Source: CAD feature listing. Evaluate the final solid. Frame: model axes, mm. A direction names the side the tool comes from. Coordinates: 2 decimals unless noted, no trailing zeros. Order: outer loops, then holes, each group sorted by start corner. A loop starts at its lowest first (then second) coordinate and runs counter-clockwise, first axis right, second up.
```python
from build123d import *

# Parameters (mm, degrees)
GEH_USEKORPUS_DEPTH                = 12.5
GEH_USEAUSH_HLUNG_DEPTH            = 10.5
PLATINENHALTERUNG_DEPTH            = 4.7
SKETCH8_R                          = 1.1
SCHRAUBL_CHER_DEPTH                = 43.096199353
SCHRAUBENMUTTER_AUSNEHMUNGEN_DEPTH = 3
SKETCH10_R                         = 3.25
SKETCH10_R_2                       = 2
BUTTON_AUSNEHMUNGEN_DEPTH          = 3
SCHNITT_LINEAR_AUSTRAGEN1_DEPTH    = 10
SKIZZE2_W                          = 52.65
SKIZZE2_H                          = 1.75
SCHNITT_LINEAR_AUSTRAGEN2_DEPTH    = 1.5
SKIZZE3_W                          = 6
SKIZZE3_H                          = 1
SCHNITT_LINEAR_AUSTRAGEN3_DEPTH    = 1.5
VERRUNDUNG1_R                      = 0.5
VERRUNDUNG2_R                      = 1


with BuildPart() as part:
    # Sketch1 → Gehäusekorpus (new body)
    with BuildSketch(Plane.XY):
        with BuildLine():
            Line((-27, -29.5), (27, -29.5))
            ThreePointArc((27, -29.5), (28.414213562, -28.914213562), (29, -27.5))
            Line((29, -27.5), (29, 27.5))
            ThreePointArc((29, 27.5), (28.414213562, 28.914213562), (27, 29.5))
            Line((27, 29.5), (-27, 29.5))
            ThreePointArc((-27, 29.5), (-28.414213562, 28.914213562), (-29, 27.5))
            Line((-29, 27.5), (-29, -27.5))
            ThreePointArc((-29, -27.5), (-28.414213562, -28.914213562), (-27, -29.5))
        make_face()
    extrude(amount=GEH_USEKORPUS_DEPTH)

    # Sketch3 → Gehäuseaushöhlung (cut)
    with BuildSketch(Plane.XY.offset(12.5)):
        with BuildLine():
            Line((-25.1, 26.5), (21.721325798, 26.5))
            ThreePointArc((21.721325798, 26.5), (22.441099985, 22.863363374), (26.1, 22.266998125))
            Line((26.1, 22.266998125), (26.1, -25.5))
            ThreePointArc((26.1, -25.5), (25.807106781, -26.207106781), (25.1, -26.5))
            Line((25.1, -26.5), (-21.721325798, -26.5))
            ThreePointArc((-21.721325798, -26.5), (-22.441099985, -22.863363374), (-26.1, -22.266998125))
            Line((-26.1, -22.266998125), (-26.1, 2.3))
            ThreePointArc((-26.1, 2.3), (-26.246446609, 2.653553391), (-26.6, 2.8))
            Line((-26.6, 2.8), (-27.1, 2.8))
            ThreePointArc((-27.1, 2.8), (-27.807106781, 3.092893219), (-28.1, 3.8))
            Line((-28.1, 3.8), (-28.1, 11.8))
            ThreePointArc((-28.1, 11.8), (-27.807106781, 12.507106781), (-27.1, 12.8))
            Line((-27.1, 12.8), (-26.6, 12.8))
            ThreePointArc((-26.6, 12.8), (-26.246446609, 12.946446609), (-26.1, 13.3))
            Line((-26.1, 13.3), (-26.1, 25.5))
            ThreePointArc((-26.1, 25.5), (-25.807106781, 26.207106781), (-25.1, 26.5))
        make_face()
    extrude(amount=-GEH_USEAUSH_HLUNG_DEPTH, mode=Mode.SUBTRACT)

    # Sketch4 → Platinenhalterung (cut)
    with BuildSketch(Plane.XY.offset(12.5)):
        with BuildLine():
            Line((-26.35, 27.75), (26.35, 27.75))
            ThreePointArc((26.35, 27.75), (27.057106781, 27.457106781), (27.35, 26.75))
            Line((27.35, 26.75), (27.35, -26.75))
            ThreePointArc((27.35, -26.75), (27.057106781, -27.457106781), (26.35, -27.75))
            Line((26.35, -27.75), (-26.35, -27.75))
            ThreePointArc((-26.35, -27.75), (-27.057106781, -27.457106781), (-27.35, -26.75))
            Line((-27.35, -26.75), (-27.35, 26.75))
            ThreePointArc((-27.35, 26.75), (-27.057106781, 27.457106781), (-26.35, 27.75))
        make_face()
    extrude(amount=-PLATINENHALTERUNG_DEPTH, mode=Mode.SUBTRACT)

    # Sketch8 → Schraublöcher (cut, through all)
    with BuildSketch(Plane.XY.offset(7.8)):
        with Locations((-24.7, -25.2)):
            Circle(SKETCH8_R)
        with Locations((24.7, 25.2)):
            Circle(SKETCH8_R)
    extrude(amount=-SCHRAUBL_CHER_DEPTH, mode=Mode.SUBTRACT)

    # Sketch9 → Schraubenmutter_Ausnehmungen (cut)
    with BuildSketch(Plane.XY):
        Polygon((27.182606158, 25.2), (25.941303079, 27.35), (23.458696921, 27.35), (22.217393842, 25.2), (23.458696921, 23.05), (25.941303079, 23.05), align=None)
        Polygon((-22.217393842, -25.2), (-23.458696921, -23.05), (-25.941303079, -23.05), (-27.182606158, -25.2), (-25.941303079, -27.35), (-23.458696921, -27.35), align=None)
    extrude(amount=SCHRAUBENMUTTER_AUSNEHMUNGEN_DEPTH, mode=Mode.SUBTRACT)

    # Sketch10 → Button_Ausnehmungen (cut)
    with BuildSketch(Plane.XZ.offset(29.5)):
        with Locations((-8, 12.5)):
            Circle(SKETCH10_R)
        with Locations((3, 12.5)):
            Circle(SKETCH10_R)
        with Locations((14, 12.5)):
            Circle(SKETCH10_R)
        with Locations((-17.8, 12.5)):
            Circle(SKETCH10_R_2)
    extrude(amount=-BUTTON_AUSNEHMUNGEN_DEPTH, mode=Mode.SUBTRACT)

    # Skizze1 → Schnitt-Linear austragen1 (cut)
    with BuildSketch(Plane(origin=(0, 29.5, 0), x_dir=(1, 0, 0), z_dir=(0, 1, 0))):
        with BuildLine():
            Line((-15.1, -12.5), (-25.6, -12.5))
            Line((-25.6, -12.5), (-25.6, -10.5))
            ThreePointArc((-25.6, -10.5), (-25.307106781, -9.792893219), (-24.6, -9.5))
            Line((-24.6, -9.5), (-16.1, -9.5))
            ThreePointArc((-16.1, -9.5), (-15.392893219, -9.792893219), (-15.1, -10.5))
            Line((-15.1, -10.5), (-15.1, -12.5))
        make_face()
        with BuildLine():
            Line((-12.1, -12.5), (-1.6, -12.5))
            Line((-1.6, -12.5), (-1.6, -10))
            ThreePointArc((-1.6, -10), (-1.746446609, -9.646446609), (-2.1, -9.5))
            Line((-2.1, -9.5), (-11.6, -9.5))
            ThreePointArc((-11.6, -9.5), (-11.953553391, -9.646446609), (-12.1, -10))
            Line((-12.1, -10), (-12.1, -12.5))
        make_face()
    extrude(amount=-SCHNITT_LINEAR_AUSTRAGEN1_DEPTH, mode=Mode.SUBTRACT)

    # Skizze2 → Schnitt-Linear austragen2 (cut)
    with BuildSketch(Plane.XY.offset(12.5)):
        with Locations((0.025, 28.625)):
            Rectangle(SKIZZE2_W, SKIZZE2_H)
    extrude(amount=-SCHNITT_LINEAR_AUSTRAGEN2_DEPTH, mode=Mode.SUBTRACT)

    # Skizze3 → Schnitt-Linear austragen3 (cut)
    with BuildSketch(Plane.XY.offset(11)):
        with Locations((2.55, 28.25)):
            Rectangle(SKIZZE3_W, SKIZZE3_H)
        with Locations((10.35, 28.25)):
            Rectangle(SKIZZE3_W, SKIZZE3_H)
    extrude(amount=-SCHNITT_LINEAR_AUSTRAGEN3_DEPTH, mode=Mode.SUBTRACT)

    # Verrundung1
    verrundung1_edges = [part.edges().sort_by_distance(p)[0] for p in [
        (-0.45, 28.25, 9.5),
        (2.55, 28.75, 9.5),
        (-0.45, 28.75, 10.25),
        (5.55, 28.25, 9.5),
        (5.55, 28.75, 10.25),
        (7.35, 28.25, 9.5),
        (10.35, 28.75, 9.5),
        (7.35, 28.75, 10.25),
        (13.35, 28.25, 9.5),
        (13.35, 28.75, 10.25),
    ]]
    fillet(verrundung1_edges, radius=VERRUNDUNG1_R)

    # Verrundung2
    verrundung2_edges = [part.edges().sort_by_distance(p)[0] for p in [
        (-22.441099985, -22.863363374, 2),
        (-26.1, -9.983499062, 2),
        (-26.246446609, 2.653553391, 2),
        (-26.85, 2.8, 2),
        (-27.807106781, 3.092893219, 2),
        (-28.1, 7.8, 2),
        (-27.807106781, 12.507106781, 2),
        (-26.85, 12.8, 2),
        (-26.246446609, 12.946446609, 2),
        (-26.1, 19.4, 2),
        (-25.807106781, 26.207106781, 2),
        (-1.689337101, 26.5, 2),
        (22.441099985, 22.863363374, 2),
        (26.1, -1.616500938, 2),
        (25.807106781, -26.207106781, 2),
        (1.689337101, -26.5, 2),
    ]]
    fillet(verrundung2_edges, radius=VERRUNDUNG2_R)


solid = part.part
```
1. Draft query along X for faces 6 (the face through (-28.43, -28.9, 6.16)), 7 (the face through (-1, 0, 2)), 8 (the face through (0, 29.5, 5)), 9 (the face through (26, 26, 3)). Return one class per face: released by +X, released by -X, zero draft, split by the parting line, or undercut.
Findings:
face 6: released by -X
face 7: undercut
face 8: zero draft
face 9: undercut
2. Ray query, line 1 (Y direction, x = 24.7, z = 5.6); line 2 (X direction, y = 24, z = 11.25); line 3 (X direction, y = -21.5, z = 5.25). Return the intervals inside material, ascending.
Findings:
line 1: y = -29.5 to -26.5, 21.95 to 24.1, 26.3 to 29.5
line 2: x = -29 to -27.35, 27.35 to 29
line 3: x = -29 to -26.1, 26.1 to 29
3. Access query for faces 1 (the face through (-23.684, -25.621, 5.434)), 2 (the face through (-26.3, 29, 12)), 3 (the face through (22.83, 24.14, 1.48)), 4 (the face through (2, -26.5, 5)), 5 (the face through (-14, -29, 12.5)). Directions: +Z, -Z, +X, -X, +Y, -Y. A direction counts if a zero-diameter tool reaches every point of the face in a straight line with its end or side. Return the directions, or none.
Findings:
face 1: +Z, -Z
face 2: +Z, +Y
face 3: -Z
face 4: +Z
face 5: +Z, +X, -X, +Y, -Y
4. Section query A-A on z = 8.5. Return loops of the section in (x, y), plus the area to 3 significant figures.
Findings:
outline: (-29, -27.5) arc R2 ccw to (-27, -29.5) - (27, -29.5) arc R2 ccw to (29, -27.5) - (29, 27.5) arc R2 ccw to (27, 29.5) - (-27, 29.5) arc R2 ccw to (-29, 27.5) - close; hole (-28.1, 3.8) arc R1 ccw to (-27.35, 2.83) - (-27.35, -26.75) arc R1 ccw to (-26.35, -27.75) - (26.35, -27.75) arc R1 ccw to (27.35, -26.75) - (27.35, 26.75) arc R1 ccw to (26.35, 27.75) - (-26.35, 27.75) arc R1 ccw to (-27.35, 26.75) - (-27.35, 12.77) arc R1 ccw to (-28.1, 11.8) - close
area: 376 mm2
5. Section query C-C on x = 3. Return loops of the section in (y, z), plus the area to 3 significant figures.
Findings:
outline: (-29.5, 0) - (29.5, 0) - (29.5, 11) - (28.75, 11) - (28.75, 10) arc R0.5 cw to (28.25, 9.5) - (27.75, 9.5) - (27.75, 7.8) - (26.5, 7.8) - (26.5, 3) arc R1 cw to (25.5, 2) - (-25.5, 2) arc R1 cw to (-26.5, 3) - (-26.5, 7.8) - (-27.75, 7.8) - (-27.75, 9.25) - (-29.5, 9.25) - close
area: 160 mm2
6. Section query D-D on y = 4.5. Return loops of the section in (x, z), plus the area to 3 significant figures.
Findings:
outline: (-29, 0) - (29, 0) - (29, 12.5) - (27.35, 12.5) - (27.35, 7.8) - (26.1, 7.8) - (26.1, 3) arc R1 cw to (25.1, 2) - (-27.1, 2) arc R1 cw to (-28.1, 3) - (-28.1, 12.5) - (-29, 12.5) - close
area: 150 mm2
7. Pin query (flat end, axial travel): P1, Ø6, axis at x = -12.5, y = 12, coming from the +Z side; P2, Ø1.9, axis at x = -13.5, y = 28.5, coming from the +Z side; P3, Ø1.4, axis at x = -19, y = 28.5, coming from the +Z side. Return the tip coordinate at first contact, or that it passes through.
Findings:
P1: stops at z = 2
P2: stops at z = 11
P3: stops at z = 9.5
8. Section query B-B on y = -9.5. Return loops of the section in (x, z).
Findings:
outline: (-29, 0) - (29, 0) - (29, 12.5) - (27.35, 12.5) - (27.35, 7.8) - (26.1, 7.8) - (26.1, 3) arc R1 cw to (25.1, 2) - (-25.1, 2) arc R1 cw to (-26.1, 3) - (-26.1, 7.8) - (-27.35, 7.8) - (-27.35, 12.5) - (-29, 12.5) - close
